Geometry check sheet. Reference: the model listing, model coordinates, mm. A direction names the side the tool comes from. Coordinates: 2 decimals unless noted, no trailing zeros. Write each loop counter-clockwise with the first axis right and the second up, starting at its lowest first coordinate (ties: lowest second). Pieces come first, ordered by that corner, then holes.
from build123d import *

# Parameters (mm, degrees)
F1_DEPTH = 5
F2_W     = 5
F2_H     = 5
F3_DEPTH = 10
F5_D     = 5


with BuildPart() as f1:
    # F0 (on Top) → F1 (new body)
    with BuildSketch(Plane.XY):
        Polygon((-15, -15), (15, -15), (15, -5), (-5, -5), (-5, 15), (-15, 15), align=None)
    extrude(amount=F1_DEPTH)

    # F2 (on face) → F3 (join)
    with BuildSketch(Plane.XY.offset(5)):
        with Locations((-12.5, -12.5)):
            Rectangle(F2_W, F2_H)
    extrude(amount=F3_DEPTH)

    # F5 (through all)
    with Locations(Plane.XY.offset(5)):
        with Locations((-10, 10)):
            Hole(F5_D / 2)


solid = f1.part
1. Sectioned sample at D-D, the plane z = 5.75. Record the boundary of the cut face in (x, y).
Computed values:
outline: (-15, -15) - (-10, -15) - (-10, -10) - (-15, -10) - close
2. Gauge pin test, flat ends, axial feed: pin 1 Ø9 at (x, y) = (-3, 4.5) entering from +Z; pin 2 Ø2.5 at (x, z) = (-13, 12) entering from +Y; pin 3 Ø4 at (y, z) = (-13.5, 10) entering from +X. Record the tip position at first contact, or that the pin passes through.
Computed values:
pin 1: stops at z = 5
pin 2: stops at y = -10
pin 3: stops at x = -10
3. Thickness scan on line 1 along Y through (x, z) = (-10, 2.9); line 2 along Y through (x, z) = (-11, 9); line 3 along Z through (x, y) = (7.75, -10.25). Record the ranges inside material, lowest first.
Computed values:
line 1: y = -15 to 7.5, 12.5 to 15
line 2: y = -15 to -10
line 3: z = 0 to 5
4. Draft check along X on faces 4 (the flat face through (-13, -10, 10)), 5 (the flat face through (-15, -4, 4)), 6 (the cylindrical face through (-9.46, 7.56, 2.47)), 7 (the flat face through (-5, 5, 2)). Enter one of: released by +X, released by -X, zero draft, split by the parting line, or undercut.
Computed values:
face 4: zero draft
face 5: released by -X
face 6: undercut
face 7: released by +X
5. Access from +Z, -Z, +X, -X, +Y, -Y to the whole of each face (thin tool, end or side, straight path). Record for faces 1 (the flat face through (15, -10, 2)), 2 (the flat face through (-10, -13, 10)), 3 (the flat face through (5, -5, 2)).
Computed values:
face 1: +Z, -Z, +X, +Y, -Y
face 2: +Z, +X, +Y, -Y
face 3: +Z, -Z, +X, +Y
6. Sectioned sample at A-A, the plane y = 10. Record the boundary of the cut face in (x, z), and give its area (3 significant figures).
Computed values:
outline: (-15, 0) - (-12.5, 0) - (-12.5, 5) - (-15, 5) - close; (-7.5, 0) - (-5, 0) - (-5, 5) - (-7.5, 5) - close
area: 25.0 mm2
7. Sectioned sample at C-C, the plane y = -10.75. Record the boundary of the cut face in (x, z).
Computed values:
outline: (-15, 0) - (15, 0) - (15, 5) - (-10, 5) - (-10, 15) - (-15, 15) - close
8. Sectioned sample at B-B, the plane z = 2.25. Record the boundary of the cut face in (x, y), and give its area (3 significant figures).
Computed values:
outline: (-15, -15) - (15, -15) - (15, -5) - (-5, -5) - (-5, 15) - (-15, 15) - close; hole circle Ø5 at (-10, 10)
area: 480 mm2
